For this review, take the finished solid that the model builds, in its own axes (mm). A direction names the side the tool comes from. Give positions to 0.01 mm unless a question says otherwise; leave off trailing zeros. Write each loop counter-clockwise with the first axis right and the second up, starting at its lowest first coordinate (ties: lowest second). Pieces come first, ordered by that corner, then holes. Notation, with made-up numbers: M 19.5,-34.75 L 40.5,-34.75 A11 ccw 40.5,-13.75 Z; hole C 36,19.5 d10. An arc over 180 degrees is marked long. Use one line per item in the form item = value. Start each with the question number.
Q1. Mouldability with a two-part tool opening along Z and no side actions: class faces 4 (the flat face through (-22, 2, 7)), 5 (the flat face through (35, 1, 4)) as released by +Z, released by -Z, zero draft, split by the parting line, or undercut.
Q2. Tool access review of faces 1 (the flat face through (14.5, 2, -24)), 2 (the flat face through (22, 2, 0)), 3 (the flat face through (0, 3, 6)): name each direction out of +Z, -Z, +X, -X, +Y, -Y from which nothing blocks a thin tool from reaching the whole face with its end or side.
Q3. Clearance check with flat-ended pins moving along their axes: pin 1 Ø1.6 at (x, y) = (22, 2) entering from -Z; pin 2 Ø3 at (x, z) = (0, -7) entering from +Y; pin 3 Ø1.5 at (y, z) = (2, -23.5) entering from +X. State where each tip first meets the part, or that it passes through.
Q4. Consider section C-C on x = -28. Write out the cut boundary in (y, z), and give its area (3 significant figures).
Q5. Consider section B-B on x = 0. Write out the cut boundary in (y, z), and give its area (3 significant figures).
Q6. Consider section A-A on z = -9.5. Write out the cut boundary in (x, y), and give its area (3 significant figures).
Q7. For probe 1 along X at (y, z) = (1.15, -3); probe 2 along X at (y, z) = (1, -7); probe 3 along Z at (x, y) = (31, 2.05), list the stretches that pass through material, from the lowest coordinate up. Write a range as [from, to].
Q8. Consider section D-D on x = -9.5. Write out the cut boundary in (y, z).
```python
from build123d import *

# Parameters (mm, degrees)
SKETCH_1_W          = 70
SKETCH_1_H          = 56
EXTRUDE_1_DEPTH     = 3
CUT_EXTRUDE_1_REACH = 46.922
SKETCH_2_R          = 1.25
SKETCH_2_W          = 23
SKETCH_2_H          = 13
SKETCH_2_W_2        = 6
SKETCH_2_H_2        = 20
SKETCH_2_W_3        = 2
SKETCH_2_H_3        = 4
SKETCH_2_W_4        = 20.5
SKETCH_2_H_4        = 7


with BuildPart() as part:
    # 草图1 → 凸台-拉伸1 (new body)
    with BuildSketch(Plane(origin=(0, 0, 0), x_dir=(1, 0, 0), z_dir=(0, 1, 0))):
        Rectangle(SKETCH_1_W, SKETCH_1_H)
    extrude(amount=EXTRUDE_1_DEPTH)

    # 草图2 → 切除-拉伸1 (cut, up to next)
    with BuildSketch(Plane(origin=(0, 3, 0), x_dir=(1, 0, 0), z_dir=(0, 1, 0)), mode=Mode.PRIVATE) as cut_extrude_1_sk1:
        with Locations(Location((0, 7, 0), (0, 0, 270))):
            Circle(SKETCH_2_R)
    cut_extrude_1_tool1 = extrude(cut_extrude_1_sk1.sketch, amount=-CUT_EXTRUDE_1_REACH, mode=Mode.PRIVATE) & part.part
    # 草图2 → 切除-拉伸1 (cut, up to next)
    with BuildSketch(Plane(origin=(0, 3, 0), x_dir=(1, 0, 0), z_dir=(0, 1, 0)), mode=Mode.PRIVATE) as cut_extrude_1_sk2:
        with Locations(Location((0, -23, 0), (0, 0, 270))):
            Circle(SKETCH_2_R)
    cut_extrude_1_tool2 = extrude(cut_extrude_1_sk2.sketch, amount=-CUT_EXTRUDE_1_REACH, mode=Mode.PRIVATE) & part.part
    # 草图2 → 切除-拉伸1 (cut, up to next)
    with BuildSketch(Plane(origin=(0, 3, 0), x_dir=(1, 0, 0), z_dir=(0, 1, 0)), mode=Mode.PRIVATE) as cut_extrude_1_sk3:
        with Locations((0, 18.5)):
            Rectangle(SKETCH_2_W, SKETCH_2_H)
    cut_extrude_1_tool3 = extrude(cut_extrude_1_sk3.sketch, amount=-CUT_EXTRUDE_1_REACH, mode=Mode.PRIVATE) & part.part
    # 草图2 → 切除-拉伸1 (cut, up to next)
    with BuildSketch(Plane(origin=(0, 3, 0), x_dir=(1, 0, 0), z_dir=(0, 1, 0)), mode=Mode.PRIVATE) as cut_extrude_1_sk4:
        with Locations((-29, -15)):
            Rectangle(SKETCH_2_W_2, SKETCH_2_H_2)
    cut_extrude_1_tool4 = extrude(cut_extrude_1_sk4.sketch, amount=-CUT_EXTRUDE_1_REACH, mode=Mode.PRIVATE) & part.part
    # 草图2 → 切除-拉伸1 (cut, up to next)
    with BuildSketch(Plane(origin=(0, 3, 0), x_dir=(1, 0, 0), z_dir=(0, 1, 0)), mode=Mode.PRIVATE) as cut_extrude_1_sk5:
        with Locations((-29, 8)):
            Rectangle(SKETCH_2_W_2, SKETCH_2_H_2)
    cut_extrude_1_tool5 = extrude(cut_extrude_1_sk5.sketch, amount=-CUT_EXTRUDE_1_REACH, mode=Mode.PRIVATE) & part.part
    # 草图2 → 切除-拉伸1 (cut, up to next)
    with BuildSketch(Plane(origin=(0, 3, 0), x_dir=(1, 0, 0), z_dir=(0, 1, 0)), mode=Mode.PRIVATE) as cut_extrude_1_sk6:
        with Locations((29, -15)):
            Rectangle(SKETCH_2_W_2, SKETCH_2_H_2)
    cut_extrude_1_tool6 = extrude(cut_extrude_1_sk6.sketch, amount=-CUT_EXTRUDE_1_REACH, mode=Mode.PRIVATE) & part.part
    # 草图2 → 切除-拉伸1 (cut, up to next)
    with BuildSketch(Plane(origin=(0, 3, 0), x_dir=(1, 0, 0), z_dir=(0, 1, 0)), mode=Mode.PRIVATE) as cut_extrude_1_sk7:
        with Locations((29, 8)):
            Rectangle(SKETCH_2_W_2, SKETCH_2_H_2)
    cut_extrude_1_tool7 = extrude(cut_extrude_1_sk7.sketch, amount=-CUT_EXTRUDE_1_REACH, mode=Mode.PRIVATE) & part.part
    # 草图2 → 切除-拉伸1 (cut, up to next)
    with BuildSketch(Plane(origin=(0, 3, 0), x_dir=(1, 0, 0), z_dir=(0, 1, 0)), mode=Mode.PRIVATE) as cut_extrude_1_sk8:
        with Locations((-22, 2)):
            Rectangle(SKETCH_2_W_3, SKETCH_2_H_3)
    cut_extrude_1_tool8 = extrude(cut_extrude_1_sk8.sketch, amount=-CUT_EXTRUDE_1_REACH, mode=Mode.PRIVATE) & part.part
    # 草图2 → 切除-拉伸1 (cut, up to next)
    with BuildSketch(Plane(origin=(0, 3, 0), x_dir=(1, 0, 0), z_dir=(0, 1, 0)), mode=Mode.PRIVATE) as cut_extrude_1_sk9:
        with Locations((-22, 14)):
            Rectangle(SKETCH_2_W_3, SKETCH_2_H_3)
    cut_extrude_1_tool9 = extrude(cut_extrude_1_sk9.sketch, amount=-CUT_EXTRUDE_1_REACH, mode=Mode.PRIVATE) & part.part
    # 草图2 → 切除-拉伸1 (cut, up to next)
    with BuildSketch(Plane(origin=(0, 3, 0), x_dir=(1, 0, 0), z_dir=(0, 1, 0)), mode=Mode.PRIVATE) as cut_extrude_1_sk10:
        with Locations((22, 2)):
            Rectangle(SKETCH_2_W_3, SKETCH_2_H_3)
    cut_extrude_1_tool10 = extrude(cut_extrude_1_sk10.sketch, amount=-CUT_EXTRUDE_1_REACH, mode=Mode.PRIVATE) & part.part
    # 草图2 → 切除-拉伸1 (cut, up to next)
    with BuildSketch(Plane(origin=(0, 3, 0), x_dir=(1, 0, 0), z_dir=(0, 1, 0)), mode=Mode.PRIVATE) as cut_extrude_1_sk11:
        with Locations((22, 14)):
            Rectangle(SKETCH_2_W_3, SKETCH_2_H_3)
    cut_extrude_1_tool11 = extrude(cut_extrude_1_sk11.sketch, amount=-CUT_EXTRUDE_1_REACH, mode=Mode.PRIVATE) & part.part
    # 草图2 → 切除-拉伸1 (cut, up to next)
    with BuildSketch(Plane(origin=(0, 3, 0), x_dir=(1, 0, 0), z_dir=(0, 1, 0)), mode=Mode.PRIVATE) as cut_extrude_1_sk12:
        with Locations((24.75, 24.5)):
            Rectangle(SKETCH_2_W_4, SKETCH_2_H_4)
    cut_extrude_1_tool12 = extrude(cut_extrude_1_sk12.sketch, amount=-CUT_EXTRUDE_1_REACH, mode=Mode.PRIVATE) & part.part
    # 草图2 → 切除-拉伸1 (cut, up to next)
    with BuildSketch(Plane(origin=(0, 3, 0), x_dir=(1, 0, 0), z_dir=(0, 1, 0)), mode=Mode.PRIVATE) as cut_extrude_1_sk13:
        with Locations((-24.75, 24.5)):
            Rectangle(SKETCH_2_W_4, SKETCH_2_H_4)
    cut_extrude_1_tool13 = extrude(cut_extrude_1_sk13.sketch, amount=-CUT_EXTRUDE_1_REACH, mode=Mode.PRIVATE) & part.part
    # 草图2 → 切除-拉伸1 (cut, up to next)
    with BuildSketch(Plane(origin=(0, 3, 0), x_dir=(1, 0, 0), z_dir=(0, 1, 0)), mode=Mode.PRIVATE) as cut_extrude_1_sk14:
        with Locations((-22, -9)):
            Rectangle(SKETCH_2_W_3, SKETCH_2_H_3)
    cut_extrude_1_tool14 = extrude(cut_extrude_1_sk14.sketch, amount=-CUT_EXTRUDE_1_REACH, mode=Mode.PRIVATE) & part.part
    # 草图2 → 切除-拉伸1 (cut, up to next)
    with BuildSketch(Plane(origin=(0, 3, 0), x_dir=(1, 0, 0), z_dir=(0, 1, 0)), mode=Mode.PRIVATE) as cut_extrude_1_sk15:
        with Locations((-22, -21)):
            Rectangle(SKETCH_2_W_3, SKETCH_2_H_3)
    cut_extrude_1_tool15 = extrude(cut_extrude_1_sk15.sketch, amount=-CUT_EXTRUDE_1_REACH, mode=Mode.PRIVATE) & part.part
    # 草图2 → 切除-拉伸1 (cut, up to next)
    with BuildSketch(Plane(origin=(0, 3, 0), x_dir=(1, 0, 0), z_dir=(0, 1, 0)), mode=Mode.PRIVATE) as cut_extrude_1_sk16:
        with Locations((22, -21)):
            Rectangle(SKETCH_2_W_3, SKETCH_2_H_3)
    cut_extrude_1_tool16 = extrude(cut_extrude_1_sk16.sketch, amount=-CUT_EXTRUDE_1_REACH, mode=Mode.PRIVATE) & part.part
    # 草图2 → 切除-拉伸1 (cut, up to next)
    with BuildSketch(Plane(origin=(0, 3, 0), x_dir=(1, 0, 0), z_dir=(0, 1, 0)), mode=Mode.PRIVATE) as cut_extrude_1_sk17:
        with Locations((22, -9)):
            Rectangle(SKETCH_2_W_3, SKETCH_2_H_3)
    cut_extrude_1_tool17 = extrude(cut_extrude_1_sk17.sketch, amount=-CUT_EXTRUDE_1_REACH, mode=Mode.PRIVATE) & part.part
    add(cut_extrude_1_tool1.solids().sort_by_distance((0, 3, -7))[0], mode=Mode.SUBTRACT)
    add(cut_extrude_1_tool2.solids().sort_by_distance((0, 3, 23))[0], mode=Mode.SUBTRACT)
    add(cut_extrude_1_tool3.solids().sort_by_distance((0, 3, -18.5))[0], mode=Mode.SUBTRACT)
    add(cut_extrude_1_tool4.solids().sort_by_distance((-29, 3, 15))[0], mode=Mode.SUBTRACT)
    add(cut_extrude_1_tool5.solids().sort_by_distance((-29, 3, -8))[0], mode=Mode.SUBTRACT)
    add(cut_extrude_1_tool6.solids().sort_by_distance((29, 3, 15))[0], mode=Mode.SUBTRACT)
    add(cut_extrude_1_tool7.solids().sort_by_distance((29, 3, -8))[0], mode=Mode.SUBTRACT)
    add(cut_extrude_1_tool8.solids().sort_by_distance((-22, 3, -2))[0], mode=Mode.SUBTRACT)
    add(cut_extrude_1_tool9.solids().sort_by_distance((-22, 3, -14))[0], mode=Mode.SUBTRACT)
    add(cut_extrude_1_tool10.solids().sort_by_distance((22, 3, -2))[0], mode=Mode.SUBTRACT)
    add(cut_extrude_1_tool11.solids().sort_by_distance((22, 3, -14))[0], mode=Mode.SUBTRACT)
    add(cut_extrude_1_tool12.solids().sort_by_distance((24.75, 3, -24.5))[0], mode=Mode.SUBTRACT)
    add(cut_extrude_1_tool13.solids().sort_by_distance((-24.75, 3, -24.5))[0], mode=Mode.SUBTRACT)
    add(cut_extrude_1_tool14.solids().sort_by_distance((-22, 3, 9))[0], mode=Mode.SUBTRACT)
    add(cut_extrude_1_tool15.solids().sort_by_distance((-22, 3, 21))[0], mode=Mode.SUBTRACT)
    add(cut_extrude_1_tool16.solids().sort_by_distance((22, 3, 21))[0], mode=Mode.SUBTRACT)
    add(cut_extrude_1_tool17.solids().sort_by_distance((22, 3, 9))[0], mode=Mode.SUBTRACT)


solid = part.part
```
Working result:
q1.face_4 = undercut
q1.face_5 = zero draft
q2.face_1 = -Z, +X, +Y, -Y
q2.face_2 = +Y, -Y
q2.face_3 = +Z, -Z, +X, -X, +Y
q3.pin_1 = -21
q3.pin_2 = 3
q3.pin_3 = 14.5
q4.outline = M 0,-21 L 3,-21 L 3,-18 L 0,-18 Z; M 0,2 L 3,2 L 3,5 L 0,5 Z; M 0,25 L 3,25 L 3,28 L 0,28 Z
q4.area = 27.0 mm²
q5.outline = M 0,-28 L 3,-28 L 3,-25 L 0,-25 Z; M 0,-12 L 3,-12 L 3,-8.25 L 0,-8.25 Z; M 0,-5.75 L 3,-5.75 L 3,21.75 L 0,21.75 Z; M 0,24.25 L 3,24.25 L 3,28 L 0,28 Z
q5.area = 114 mm²
q6.outline = M -35,0 L -32,0 L -32,3 L -35,3 Z; M -26,0 L 26,0 L 26,3 L -26,3 Z; M 32,0 L 35,0 L 35,3 L 32,3 Z
q6.area = 174 mm²
q7.probe_1 = [-35, -32], [-26, -23], [-21, 21], [23, 26], [32, 35]
q7.probe_2 = [-35, -32], [-26, -1.25], [1.25, 26], [32, 35]
q7.probe_3 = [-21, -18], [2, 5], [25, 28]
q8.outline = M 0,-28 L 3,-28 L 3,-25 L 0,-25 Z; M 0,-12 L 3,-12 L 3,28 L 0,28 Z
